Geometry: final body of the model. Coordinates: model frame, mm. Face numbers are marked on the shaded views. A direction names the side the tool comes from. Coordinates: 2 decimals unless noted, no trailing zeros. Order: outer loops, then holes, each group sorted by start corner. A loop starts at its lowest first (then second) coordinate and runs counter-clockwise, first axis right, second up. Notation, with made-up numbers: (55, 33) -> (85, 33) arc R7 ccw to (85, 43) -> close; hole circle Ø8 at (48.5, 63.25). An arc over 180 degrees is marked (long way). Answer in a Markdown table with one row per item. Add a question column.
1) Ray query, line 1 (X direction, y = 1.55, z = 0); line 2 (X direction, y = 3, z = 0); line 3 (Y direction, x = 7, z = 0.5). Return the intervals inside material, ascending. Write a range as from..to.
2) Section query A-A on x = 0. Return the cut outline in (y, z).
3) Contact query for flat-ended pins moving along their axis: P1, Ø8, axis at x = -2, z = 3.5, coming from the -Y side; P2, Ø1.2, axis at x = 10, z = 0, coming from the -Y side; P3, Ø7, axis at x = 0, z = -2, coming from the +Y side; P4, Ø1.5, axis at y = 1, z = -5, coming from the +X side. Output: stop coordinate, or through.
4) Section query C-C on y = 0.4. Return the cut outline in (x, z).
5) Pull-direction query (Z, two-part tool) for the marked faces 1, 2, 3 and 4; classes: +Z half, -Z half, draft (parallel to the pull), parting line (faces both ways), or undercut.
6) Set-up query: the marked faces 5 and 6. Return all of +Z, -Z, +X, -X, +Y, -Y with unobstructed straight access to the full face (end or side cutting, diameter ignored); none if empty.
7) Section query B-B on z = 0. Return the cut outline in (x, y).
8) Section query D-D on z = -3.25. Return the cut outline in (x, y).
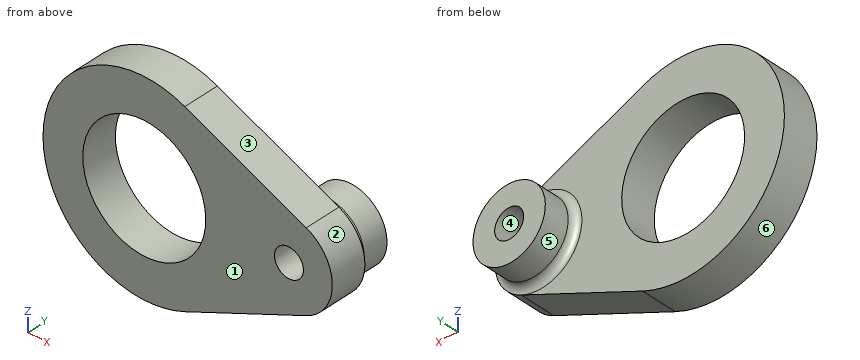
```python
from build123d import *

# Parameters (mm, degrees)
SKETCH_1_R      = 7
SKETCH_1_R_2    = 4.2499999999999964
SKETCH_1_R_3    = 0.9999999999999998
EXTRUDE_1_DEPTH = 2.5
SKETCH_2_R      = 2.5000000000000004
SKETCH_2_R_2    = 0.9999999999999998
EXTRUDE_2_DEPTH = 2.25


with BuildPart() as part:
    # 草图1 → 凸台-拉伸1 (new body)
    # profile 1 of 2: a face of its own
    with BuildSketch(Plane(origin=(0, 0, 0), x_dir=(1, 0, 0), z_dir=(0, 1, 0))):
        Circle(SKETCH_1_R)
        with Locations(Location((0, 0, 0), (0, 0, 270))):
            Circle(SKETCH_1_R_2, mode=Mode.SUBTRACT)
    # profile 2 of 2: a face of its own
    with BuildSketch(Plane(origin=(0, 0, 0), x_dir=(1, 0, 0), z_dir=(0, 1, 0))):
        with BuildLine():
            Line((11.2, 2.749545416973503), (2.8000000000000003, 6.415605972938175))
            ThreePointArc((2.8000000000000007, 6.415605972938176), (5.856620185738529, 3.8340579025361627), (7, 0))
            ThreePointArc((7, -1.71e-15), (5.856620185738526, -3.834057902536167), (2.799999999999998, -6.4156059729381765))
            Line((2.8000000000000007, -6.415605972938176), (11.2, -2.749545416973503))
            ThreePointArc((11.2, -2.749545416973503), (13, 0), (11.2, 2.7495454169735036))
        make_face()
        with Locations(Location((10, 0, 0), (0, 0, 270))):
            Circle(SKETCH_1_R_3, mode=Mode.SUBTRACT)
    extrude(amount=EXTRUDE_1_DEPTH)

    # 草图2 → 凸台-拉伸2 (add)
    with BuildSketch(Plane(origin=(0, 2.5, 0), x_dir=(1, 0, 0), z_dir=(0, 1, 0))):
        with Locations(Location((10, 0, 0), (0, 0, 270))):
            Circle(SKETCH_2_R)
        with Locations(Location((10, 0, 0), (0, 0, 270))):
            Circle(SKETCH_2_R_2, mode=Mode.SUBTRACT)
    extrude(amount=EXTRUDE_2_DEPTH)

    # 圆角2: read off the stored shape, not the designer's step
    # 圆角2 outline → 圆角2 (revolve)
    with BuildSketch(Plane(origin=(10, 0, 0), x_dir=(1, 0, 0), z_dir=(0, 0, 1))):
        with BuildLine():
            ThreePointArc((3, 2.5), (2.646446609, 2.646446609), (2.5, 3))
            Line((2.5, 3), (2.5, 2.5))
            Line((2.5, 2.5), (3, 2.5))
        make_face()
    revolve(axis=Axis((10, 0, 0), (0, 1, 0)))


solid = part.part
```
Result:
| question | item | result |
|---|---|---|
| 1 | line 1 | -7..-4.25, 4.25..9, 11..13 |
| 1 | line 2 | 7.5..9, 11..12.5 |
| 1 | line 3 | 0..2.5 |
| 2 | outline | (0, -7) -> (2.5, -7) -> (2.5, -4.25) -> (0, -4.25) -> close; (0, 4.25) -> (2.5, 4.25) -> (2.5, 7) -> (0, 7) -> close |
| 3 | P1 | y = 0 |
| 3 | P2 | through |
| 3 | P3 | y = 2.5 |
| 3 | P4 | x = 7.76 |
| 4 | outline | (2.8, -6.42) -> (11.2, -2.75) arc R3 ccw to (11.2, 2.75) -> (2.8, 6.42) arc R7 ccw (long way) to start; hole circle Ø8.5 at (0, 0); hole circle Ø2 at (10, 0) |
| 5 | face 1 | draft |
| 5 | face 2 | parting line |
| 5 | face 3 | +Z half |
| 5 | face 4 | undercut |
| 6 | face 5 | +Y |
| 6 | face 6 | +Y, -Y |
| 7 | outline | (-7, 0) -> (-4.25, 0) -> (-4.25, 2.5) -> (-7, 2.5) -> close; (4.25, 0) -> (9, 0) -> (9, 4.75) -> (7.5, 4.75) -> (7.5, 3) arc R0.5 cw to (7, 2.5) -> (4.25, 2.5) -> close; (11, 0) -> (13, 0) -> (13, 2.5) arc R0.5 cw to (12.5, 3) -> (12.5, 4.75) -> (11, 4.75) -> close |
| 8 | outline | (-6.2, 0) -> (-2.74, 0) -> (-2.74, 2.5) -> (-6.2, 2.5) -> close; (2.74, 0) -> (10.05, 0) -> (10.05, 2.5) -> (2.74, 2.5) -> close |
